from build123d import *

# Parameters (mm, degrees)
BOSS_EXTRUDE1_DEPTH = 19.2532
BOSS_EXTRUDE2_START = -0.8382
SKETCH2_R           = 2.032
BOSS_EXTRUDE2_DEPTH = 0.8382
SKETCH3_R           = 4.6355
BOSS_EXTRUDE3_DEPTH = 1.8796
SKETCH4_R           = 2.4892
BOSS_EXTRUDE4_DEPTH = 8.128
CUT_EXTRUDE1_START  = -6.096
CUT_EXTRUDE1_DEPTH  = 6.096


with BuildPart() as part:
    # Sketch1 → Boss-Extrude1 (new body)
    with BuildSketch(Plane.XY):
        with BuildLine():
            Line((-7.366, -17.78), (7.366, -17.78))
            Line((7.366, -17.78), (7.366, -11.870254589))
            ThreePointArc((7.366, -11.870254589), (0, 13.97), (-7.366, -11.870254589))
            Line((-7.366, -11.870254589), (-7.366, -17.78))
        make_face()
    extrude(amount=BOSS_EXTRUDE1_DEPTH)

    # Sketch2 → Boss-Extrude2 (add)
    # profile 1 of 2: a face of its own
    with BuildSketch(Plane.XY.offset(19.2532).offset(BOSS_EXTRUDE2_START)):
        with BuildLine():
            Line((-13.52310885, -3.5052), (-17.4752, -3.5052))
            ThreePointArc((-17.4752, -3.5052), (-20.9804, 0), (-17.4752, 3.5052))
            Line((-17.4752, 3.5052), (-13.52310885, 3.5052))
            ThreePointArc((-13.52310885, 3.5052), (-13.97, 0), (-13.52310885, -3.5052))
        make_face()
        with Locations((-17.4752, 0)):
            Circle(SKETCH2_R, mode=Mode.SUBTRACT)
    # profile 2 of 2: a face of its own
    with BuildSketch(Plane.XY.offset(19.2532).offset(BOSS_EXTRUDE2_START)):
        with BuildLine():
            Line((13.52310885, 3.5052), (17.4752, 3.5052))
            ThreePointArc((17.4752, 3.5052), (20.9804, 0), (17.4752, -3.5052))
            Line((17.4752, -3.5052), (13.52310885, -3.5052))
            ThreePointArc((13.52310885, -3.5052), (13.97, 0), (13.52310885, 3.5052))
        make_face()
        with Locations(Location((17.4752, 0, 0), (0, 0, 180))):
            Circle(SKETCH2_R, mode=Mode.SUBTRACT)
    extrude(amount=BOSS_EXTRUDE2_DEPTH)

    # Sketch3 → Boss-Extrude3 (add)
    with BuildSketch(Plane.XY.offset(19.2532)):
        with Locations((0, 7.7343)):
            Circle(SKETCH3_R)
    extrude(amount=BOSS_EXTRUDE3_DEPTH)

    # Sketch4 → Boss-Extrude4 (add)
    with BuildSketch(Plane.XY.offset(21.1328)):
        with Locations((0, 7.7343)):
            Circle(SKETCH4_R)
    extrude(amount=BOSS_EXTRUDE4_DEPTH)

    # Sketch5 → Cut-Extrude1 (cut)
    with BuildSketch(Plane.XY.offset(29.2608).offset(CUT_EXTRUDE1_START)):
        with BuildLine():
            Line((-1.524, 9.702431256), (-1.524, 5.766168744))
            ThreePointArc((-1.524, 5.766168744), (-2.4892, 7.7343), (-1.524, 9.702431256))
        make_face()
        with BuildLine():
            Line((1.524, 9.702431256), (1.524, 5.766168744))
            ThreePointArc((1.524, 5.766168744), (2.4892, 7.7343), (1.524, 9.702431256))
        make_face()
    extrude(amount=CUT_EXTRUDE1_DEPTH, mode=Mode.SUBTRACT)


solid = part.part
Design review of the part built by this model. Coordinates are the model's own, in mm. A direction names the side the tool comes from. Round coordinates to 2 decimals unless told otherwise and drop trailing zeros. Write each loop counter-clockwise with the first axis right and the second up, starting at its lowest first coordinate (ties: lowest second). Pieces come first, ordered by that corner, then holes. Notation, with made-up numbers: (25, -8.5) - (56, -8.5) arc R17 ccw to (56, 5.5) - close; hole circle Ø7 at (82.5, 0.25). An arc over 180 degrees is marked (long way). Use a Markdown table: item, result. Add a question column.
1. For faces 4 (the face through (2, 6, 21.133)), 5 (the face through (-1.524, 8, 26)), 6 (the face through (0.51, 13.96, 9.49)), 7 (the face through (-7.366, -15, 9)), list the 3-axis set-ups (+Z, -Z, +X, -X, +Y, -Y) from which the entire face can be reached by the end or side of a thin tool; tool diameter is ignored.
2. We need section C-C (y = 7). State the section outline as (x, z) points.
3. Mouldability with a two-part tool opening along Y and no side actions: class faces 1 (the face through (-20.98, -0.08, 18.83)), 2 (the face through (15.537, -0.61, 18.828)), 3 (the face through (0, 8, 29.261)) as +Y half, -Y half, draft (parallel to the pull), parting line (faces both ways), or undercut.
4. We need section D-D (z = 15.5). State the section outline as (x, y) points, then the cut area to 3 significant figures.
5. We need section A-A (y = 0). State the section outline as (x, z) points (3 decimals), then the cut area to 3 significant figures.
6. Clearance check with flat-ended pins moving along their axes: pin 1 (0.7 mm diameter, centred on x = 15.5, z = 19, fed in from -Y); pin 2 (0.8 mm diameter, centred on x = -2, y = 8, fed in from +Z); pin 3 (1 mm diameter, centred on y = 3.5, z = 11, fed in from +X); pin 4 (1.1 mm diameter, centred on x = 2, y = 8.5, fed in from +Z). State where each tip first meets the part, or that it passes through.
7. Wall thickness on probe 1 along Z at (x, y) = (12, -5.5); probe 2 along Z at (x, y) = (-2.5, 11.5); probe 3 along X at (y, z) = (-16, 5.5): over which ranges is each line inside the solid? List them lowest first.
8. We need section B-B (x = 0). State the section outline as (y, z) points, then the cut area to 3 significant figures.
Output:
| question | item | result |
|---|---|---|
| 1 | face 4 | +Z |
| 1 | face 5 | +Z, -X, +Y, -Y |
| 1 | face 6 | -Z |
| 1 | face 7 | +Z, -Z, -X, -Y |
| 2 | outline | (-12.09, 0) - (12.09, 0) - (12.09, 19.25) - (4.58, 19.25) - (4.58, 21.13) - (2.38, 21.13) - (2.38, 23.16) - (1.52, 23.16) - (1.52, 29.26) - (-1.52, 29.26) - (-1.52, 23.16) - (-2.38, 23.16) - (-2.38, 21.13) - (-4.58, 21.13) - (-4.58, 19.25) - (-12.09, 19.25) - close |
| 3 | face 1 | parting line |
| 3 | face 2 | undercut |
| 3 | face 3 | draft |
| 4 | outline | (-7.37, -17.78) - (7.37, -17.78) - (7.37, -11.87) arc R13.97 ccw (long way) to (-7.37, -11.87) - close |
| 4 | area | 679 mm2 |
| 5 | outline | (-20.98, 18.415) - (-19.507, 18.415) - (-19.507, 19.253) - (-20.98, 19.253) - close; (-15.443, 18.415) - (-13.97, 18.415) - (-13.97, 0) - (13.97, 0) - (13.97, 18.415) - (15.443, 18.415) - (15.443, 19.253) - (-15.443, 19.253) - close; (19.507, 18.415) - (20.98, 18.415) - (20.98, 19.253) - (19.507, 19.253) - close |
| 5 | area | 543 mm2 |
| 6 | pin 1 | stops at y = -3.51 |
| 6 | pin 2 | stops at z = 23.16 |
| 6 | pin 3 | stops at x = 13.64 |
| 6 | pin 4 | stops at z = 29.26 |
| 7 | probe 1 | z = 0 to 19.25 |
| 7 | probe 2 | z = 0 to 21.13 |
| 7 | probe 3 | x = -7.37 to 7.37 |
| 8 | outline | (-17.78, 0) - (13.97, 0) - (13.97, 19.25) - (12.37, 19.25) - (12.37, 21.13) - (10.22, 21.13) - (10.22, 29.26) - (5.25, 29.26) - (5.25, 21.13) - (3.1, 21.13) - (3.1, 19.25) - (-17.78, 19.25) - close |
| 8 | area | 669 mm2 |
